```python
from build123d import *

# Parameters (mm, degrees)
CROQUIS1_W              = 200
CROQUIS1_H              = 40
CROQUIS1_R              = 2
SALIENTE_EXTRUIR1_DEPTH = 10
CROQUIS2_W              = 200
CROQUIS2_H              = 7
SALIENTE_EXTRUIR3_DEPTH = 20
CROQUIS3_W              = 84
CROQUIS3_H              = 26
SALIENTE_EXTRUIR4_DEPTH = 20
CROQUIS5_R              = 1.5
CORTAR_EXTRUIR1_DEPTH   = 10
CORTAR_EXTRUIR2_DEPTH   = 60
CROQUIS8_W              = 32
CROQUIS8_H              = 26
SALIENTE_EXTRUIR5_DEPTH = 20
CROQUIS7_R              = 3
CORTAR_EXTRUIR3_DEPTH   = 20


with BuildPart() as part:
    # Croquis1 → Saliente-Extruir1 (new body)
    with BuildSketch(Plane.XY):
        Rectangle(CROQUIS1_W, CROQUIS1_H)
        with Locations((0, 9.779)):
            Circle(CROQUIS1_R, mode=Mode.SUBTRACT)
        with Locations((6.914797213, 6.914797213)):
            Circle(CROQUIS1_R, mode=Mode.SUBTRACT)
        with Locations((9.779, 0)):
            Circle(CROQUIS1_R, mode=Mode.SUBTRACT)
        with Locations((6.914797213, -6.914797213)):
            Circle(CROQUIS1_R, mode=Mode.SUBTRACT)
        with Locations((0, -9.779)):
            Circle(CROQUIS1_R, mode=Mode.SUBTRACT)
        with Locations((-6.914797213, -6.914797213)):
            Circle(CROQUIS1_R, mode=Mode.SUBTRACT)
        with Locations((-9.779, 0)):
            Circle(CROQUIS1_R, mode=Mode.SUBTRACT)
        with Locations((-6.914797213, 6.914797213)):
            Circle(CROQUIS1_R, mode=Mode.SUBTRACT)
    extrude(amount=SALIENTE_EXTRUIR1_DEPTH)

    # Croquis2 → Saliente-Extruir3 (add)
    with BuildSketch(Plane.XY.offset(10)):
        with Locations((0, -16.5)):
            Rectangle(CROQUIS2_W, CROQUIS2_H)
        with Locations((0, 16.5)):
            Rectangle(CROQUIS2_W, CROQUIS2_H)
    extrude(amount=SALIENTE_EXTRUIR3_DEPTH)

    # Croquis3 → Saliente-Extruir4 (add)
    with BuildSketch(Plane.XY.offset(10)):
        with Locations((-58, 0)):
            Rectangle(CROQUIS3_W, CROQUIS3_H)
        with Locations((58, 0)):
            Rectangle(CROQUIS3_W, CROQUIS3_H)
    extrude(amount=SALIENTE_EXTRUIR4_DEPTH)

    # Croquis5 → Cortar-Extruir1 (cut)
    with BuildSketch(Plane(origin=(0, 20, 0), x_dir=(-1, 0, 0), z_dir=(0, -1, 0))):
        with Locations((-63.9, -15)):
            Circle(CROQUIS5_R)
        with Locations((-72.9, -10)):
            Circle(CROQUIS5_R)
        with Locations((-72.9, -20)):
            Circle(CROQUIS5_R)
        with Locations((-82.9, -20)):
            Circle(CROQUIS5_R)
        with Locations((-82.9, -10)):
            Circle(CROQUIS5_R)
        with Locations((-91.9, -15)):
            Circle(CROQUIS5_R)
    extrude(amount=CORTAR_EXTRUIR1_DEPTH, mode=Mode.SUBTRACT)

    # Croquis6 → Cortar-Extruir2 (cut)
    with BuildSketch(Plane.ZY.offset(100)):
        with BuildLine():
            Line((-8.93194877, 20), (-8.93194877, -20))
            Line((-8.93194877, -20), (0, -20))
            Line((0, -20), (0, -13.228756555))
            ThreePointArc((0, -13.228756555), (-5, 0), (0, 13.228756555))
            Line((0, 13.228756555), (0, 20))
            Line((0, 20), (-8.93194877, 20))
        make_face()
        with BuildLine():
            Line((30, -13.228756555), (30, -20))
            Line((30, -20), (38.93194877, -20))
            Line((38.93194877, -20), (38.93194877, 20))
            Line((38.93194877, 20), (30, 20))
            Line((30, 20), (30, 13.228756555))
            ThreePointArc((30, 13.228756555), (33.708286934, 7.071067812), (35, 0))
            ThreePointArc((35, 0), (33.708286934, -7.071067812), (30, -13.228756555))
        make_face()
        with BuildLine():
            ThreePointArc((30, -13.228756555), (23.228756555, -18.228756555), (15, -20))
            Line((15, -20), (30, -20))
            Line((30, -20), (30, -13.228756555))
        make_face()
        with BuildLine():
            Line((0, -13.228756555), (0, -20))
            Line((0, -20), (15, -20))
            ThreePointArc((15, -20), (6.771243445, -18.228756555), (0, -13.228756555))
        make_face()
        with BuildLine():
            Line((15, 20), (0, 20))
            Line((0, 20), (0, 13.228756555))
            ThreePointArc((0, 13.228756555), (6.771243445, 18.228756555), (15, 20))
        make_face()
        with BuildLine():
            Line((30, 20), (15, 20))
            ThreePointArc((15, 20), (23.228756555, 18.228756555), (30, 13.228756555))
            Line((30, 13.228756555), (30, 20))
        make_face()
    extrude(amount=-CORTAR_EXTRUIR2_DEPTH, mode=Mode.SUBTRACT)

    # Croquis8 → Saliente-Extruir5 (add)
    with BuildSketch(Plane.XY.offset(10)):
        Rectangle(CROQUIS8_W, CROQUIS8_H)
    extrude(amount=SALIENTE_EXTRUIR5_DEPTH)

    # Croquis7 → Cortar-Extruir3 (cut)
    with BuildSketch(Plane.XY.offset(10)):
        with Locations((0, 9.779)):
            Circle(CROQUIS7_R)
        with Locations((-6.914797213, 6.914797213)):
            Circle(CROQUIS7_R)
        with Locations((-9.779, 0)):
            Circle(CROQUIS7_R)
        with Locations((6.914797213, 6.914797213)):
            Circle(CROQUIS7_R)
        with Locations((9.779, 0)):
            Circle(CROQUIS7_R)
        with Locations((-6.914797213, -6.914797213)):
            Circle(CROQUIS7_R)
        with Locations((6.914797213, -6.914797213)):
            Circle(CROQUIS7_R)
        with Locations((0, -9.779)):
            Circle(CROQUIS7_R)
    extrude(amount=CORTAR_EXTRUIR3_DEPTH, mode=Mode.SUBTRACT)


solid = part.part
```
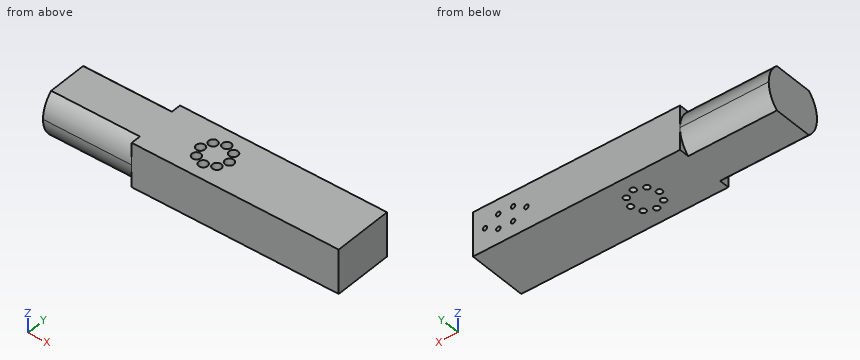
Work out the finished part from the listing and answer in its coordinate system (mm). Give positions to 0.01 mm unless a question says otherwise; leave off trailing zeros. Loops run counter-clockwise (first coordinate to the right, second up) from the corner with the lowest first, then second, coordinate; pieces in that order, holes last. Notation, with made-up numbers: M 5,-3.5 L 50,-3.5 A29 cw 50,21.5 Z; hole C 74,-34.5 d9. An arc over 180 degrees is marked long. One line per item, written item: value. Start each with the question number.
1. Each of these flat-tipped pins is pushed along its axis until it touches: P1, Ø0.9, axis at x = 64, z = 14.5, coming from the +Y side; P2, Ø3, axis at x = -6, y = -6.5, coming from the +Z side. Where does it stop, or does it pass through?
2. Find section A-A (x = 0). Give the vertices of the cut face in (y, z).
3. Find the intervals of material crossed by probe 1 along X at (y, z) = (16.75, 15); probe 2 along X at (y, z) = (16, 10); probe 3 along Y at (x, z) = (5, 12.5), in increasing order.
4. Find section D-D (x = -75). Give the vertices of the cut face in (y, z).
5. Find section B-B (y = -16). Give the vertices of the cut face in (x, z).
6. Find section C-C (z = 27.5). State how many separate pieces and enclosed holes the cut face has, and give its area (3 significant figures).
Reported:
1. P1: stops at y = 10
1. P2: stops at z = 10
2. outline: M -20,0 L -11.78,0 L -11.78,10 L -12.78,10 L -12.78,30 L -20,30 Z; M -7.78,0 L 7.78,0 L 7.78,10 L 6.78,10 L 6.78,30 L -6.78,30 L -6.78,10 L -7.78,10 Z; M 11.78,0 L 20,0 L 20,30 L 12.78,30 L 12.78,10 L 11.78,10 Z
3. probe 1: x = -100 to 62.4, 65.4 to 90.4, 93.4 to 100
3. probe 2: x = -100 to 71.4, 74.4 to 81.4, 84.4 to 100
3. probe 3: y = -20 to -9.22, -4.61 to 4.61, 9.22 to 20
4. outline: M -13.23,0 L 13.23,0 A20 ccw 13.23,30 L -13.23,30 A20 ccw Z
5. outline: M -100,3 L -40,3 L -40,0 L 100,0 L 100,30 L -40,30 L -40,27 L -100,27 Z
6. separate pieces: 1
6. enclosed holes: 8
6. area: 7,250 mm²
